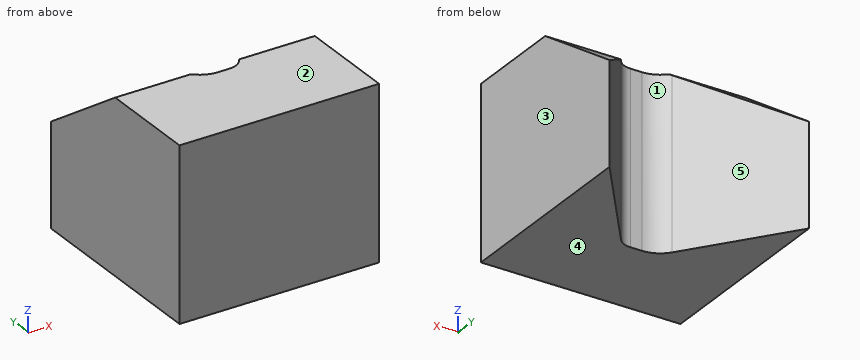
Solid Edge part; units mm, degrees
sketch "Sketch1" plane through (0, 0, 0) normal (0, 0, 1) x (1, 0, 0)
  line L0 (14.6283, 60.7642) -> (-2.8717, 37.6396)
  line L1 (-2.8717, 37.6396) -> (-20.3717, 60.7642)
  line L2 (-20.3717, 60.7642) -> (-20.3717, 25.7642)
  line L3 (-20.3717, 25.7642) -> (14.6283, 25.7642)
  line L4 (14.6283, 25.7642) -> (14.6283, 60.7642)
extrude "Protrusion1" add sketch "Sketch1" along normal blind 30
chamfer "Chamfer_1" distance 5 angle 45 1 edges at (-2.8717, 37.6396, 15)
sketch "Sketch2" plane through (14.6283, 43.2642, 15) normal (1, 0, 0) x (0, 0, -1)
  line L0 (-15, 0) -> (-15, 17.5)
  line L1 (-15, 17.5) -> (-2.9359, 17.5)
  line L2 (-15, 0) -> (-2.9359, 17.5)
extrude "ExtrudedCutout_1" cut sketch "Sketch2" against normal blind 45
fillet "Round_2" radius 5 1 edges at (-5.8889, 41.6266, 15)
fillet "Round_3" radius 3 1 edges at (0.1455, 41.6266, 15)
properties material "Chocolate"
The model under review builds one solid part; all positions refer to its coordinate system, in mm. Face numbers are marked on the shaded views. A direction names the side the tool comes from. Give positions to 0.01 mm unless a question says otherwise; leave off trailing zeros. Write each loop counter-clockwise with the first axis right and the second up, starting at its lowest first coordinate (ties: lowest second). Pieces come first, ordered by that corner, then holes. Notation, with made-up numbers: M 48,49 L 99,49 A12 ccw 99,58 Z; hole C 67.25,34 d1. An arc over 180 degrees is marked long. Write each question's results on one line, items separated by ' | '. Start each with the question number.
1. Insertion check: pin 1 Ø10 at (x, y) = (9.5, 46) entering from -Z; pin 2 Ø2.5 at (x, z) = (-2, 10.5) entering from +Y; pin 3 Ø5 at (x, z) = (-6, 17.5) entering from +Y. Each pin has a flat end and moves straight along its axis. Give the tip position at first contact, or say it passes through.
2. We need section C-C (x = 8). Write out the cut boundary in (y, z).
3. For probe 1 along X at (y, z) = (44, 19); probe 2 along X at (y, z) = (53, 17.5); probe 3 along Y at (x, z) = (3, 6), list the stretches that pass through material, from the lowest coordinate up. Write a range as [from, to].
4. We need section D-D (z = 27). Write out the cut boundary in (x, y).
5. For the marked faces 4 and 5, list the 3-axis set-ups (+Z, -Z, +X, -X, +Y, -Y) from which the entire face can be reached by the end or side of a thin tool; tool diameter is ignored.
6. We need section B-B (z = 4). Write out the cut boundary in (x, y).
7. We need section A-A (y = 56.5). Write out the cut boundary in (x, z).
8. Mouldability with a two-part tool opening along X and no side actions: class the marked faces 1, 2 and 3 as released by +X, released by -X, zero draft, split by the parting line, or undercut.
Results found:
1) pin 1: stops at z = 0 | pin 2: stops at y = 41.69 | pin 3: stops at y = 45.08
2) outline: M 25.76,0 L 52.01,0 L 52.01,23.97 L 43.26,30 L 25.76,30 Z
3) probe 1: x = [-20.37, -7.69], [1.94, 14.63] | probe 2: x = [-20.37, -14.5], [8.75, 14.63] | probe 3: y = [25.76, 45.4]
4) outline: M -20.37,25.76 L 14.63,25.76 L 14.63,47.62 L 4.68,47.62 L 1.05,42.82 A3 cw -1.35,41.63 L -3.4,41.63 A5 cw -7.39,43.61 L -10.42,47.62 L -20.37,47.62 Z
5) face 4: -Z, +X, -X, +Y, -Y | face 5: +Z, -Z, +Y
6) outline: M -20.37,25.76 L 14.63,25.76 L 14.63,60.76 L 1.05,42.82 A3 cw -1.35,41.63 L -3.4,41.63 A5 cw -7.39,43.61 L -20.37,60.76 Z
7) outline: M -20.37,0 L -17.14,0 L -17.14,20.88 L -20.37,20.88 Z; M 11.4,0 L 14.63,0 L 14.63,20.88 L 11.4,20.88 Z
8) face 1: undercut | face 2: zero draft | face 3: released by +X
